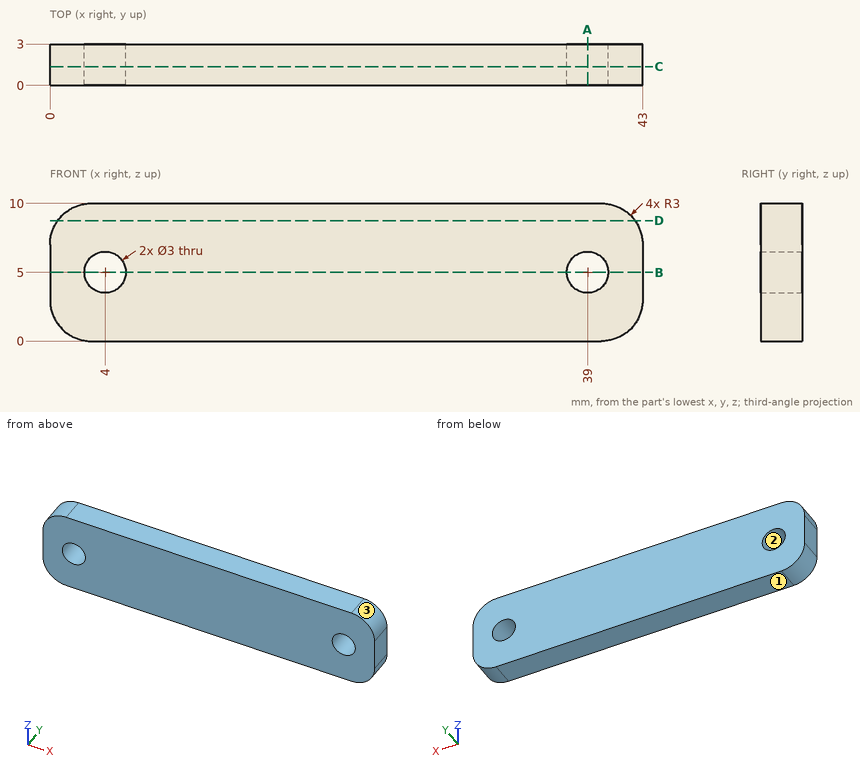
Could you check a few things on this drawing? It's one solid part, dimensions in mm from its lowest x, y, z. Give positions to 0.01 mm unless a question says otherwise; leave off trailing zeros. Order: outer loops, then holes, each group sorted by start corner. A loop starts at its lowest first (then second) coordinate and runs counter-clockwise, first axis right, second up.
1. Suppose I cut it at A-A (x = 39). Write out the boundary of the cut face in (y, z).
Answers below:
outline: (0, 0) - (3, 0) - (3, 3.5) - (0, 3.5) - close; (0, 6.5) - (3, 6.5) - (3, 10) - (0, 10) - close
2. Suppose I cut it at B-B (z = 5). Write out the boundary of the cut face in (x, y), plus the area to 3 significant figures.
Answers below:
outline: (0, 0) - (2.5, 0) - (2.5, 3) - (0, 3) - close; (5.5, 0) - (37.5, 0) - (37.5, 3) - (5.5, 3) - close; (40.5, 0) - (43, 0) - (43, 3) - (40.5, 3) - close
area: 111 mm2
3. For pin 1 (4 mm diameter, centred on x = 39, z = 5, fed in from -Y), with a flat end and sliding along its axis, tell me the tip position at first contact or that it passes through.
Answers below:
pin 1: stops at y = 0
4. Suppose I cut it at C-C (y = 1.35). Write out the boundary of the cut face in (x, z).
Answers below:
outline: (0, 3) arc R3 ccw to (3, 0) - (40, 0) arc R3 ccw to (43, 3) - (43, 7) arc R3 ccw to (40, 10) - (3, 10) arc R3 ccw to (0, 7) - close; hole circle Ø3 at (4, 5); hole circle Ø3 at (39, 5)
5. Suppose I cut it at D-D (z = 8.75). Write out the boundary of the cut face in (x, y), plus the area to 3 significant figures.
Answers below:
outline: (0.56, 0) - (42.44, 0) - (42.44, 3) - (0.56, 3) - close
area: 126 mm2
6. I need wall thicknesses on L1, parallel to X at y = 0.75, z = 5; L2, parallel to Z at x = 39, y = 1.3; L3, parallel to X at y = 0.3, z = 3.75. Which ranges of each line are inside material? Lowest first, please.
Answers below:
L1: x = 0 to 2.5, 5.5 to 37.5, 40.5 to 43
L2: z = 0 to 3.5, 6.5 to 10
L3: x = 0 to 3.17, 4.83 to 38.17, 39.83 to 43
7. Thinking about a two-plate mould opening in X: for the marked faces 1, 2 and 3, which applies, +X half, -X half, draft (parallel to the pull), parting line (faces both ways), or undercut?
Answers below:
face 1: draft
face 2: undercut
face 3: +X half
